Check sheet for the drawn part. Datum: minimum x, y, z corner. Units: mm. A direction names the side the tool comes from. Coordinates: 2 decimals unless noted, no trailing zeros. Loops run counter-clockwise (first coordinate to the right, second up) from the corner with the lowest first, then second, coordinate; pieces in that order, holes last. Notation, with made-up numbers: (84.25, 72.25) -> (103.25, 72.25) arc R23 ccw to (103.25, 101.25) -> close; hole circle Ø5 at (-12, 10.5). An arc over 180 degrees is marked (long way). Use CSV: the item, a comma, the result in double quotes. Start each with the question number.
1. Release check for a two-part mould opening along X. For the marked faces 3, 4 and 5 record: pulls with the +X half, pulls with the -X half, needs draft (parallel to the pull), parting line crosses it, or undercut.
2. Sectioned sample at D-D, the plane x = 37.5. Record the cut outline in (y, z), and give its area (3 significant figures).
3. Sectioned sample at A-A, the plane y = 35. Record the cut outline in (x, z).
4. Gauge pin test, flat ends, axial feed: pin 1 (8 mm diameter, centred on x = 9.5, z = 54, fed in from +Y); pin 2 (6 mm diameter, centred on y = 31.5, z = 45, fed in from -X). Record the tip position at first contact, or that the pin passes through.
5. Sectioned sample at B-B, the plane x = 30. Record the cut outline in (y, z), and give its area (3 significant figures).
6. Set-up check for the marked faces 1 and 2: record each of +Z, -Z, +X, -X, +Y, -Y from which the full face is reachable in a straight line by a thin tool's end or side.
7. Thickness scan on L1, parallel to X at y = 31, z = 38; L2, parallel to Z at x = 30, y = 1.5; L3, parallel to Y at x = 59.25, z = 45. Record the ranges inside material, lowest first.
8. Sectioned sample at C-C, the plane z = 50. Record the cut outline in (x, y), and give its area (3 significant figures).
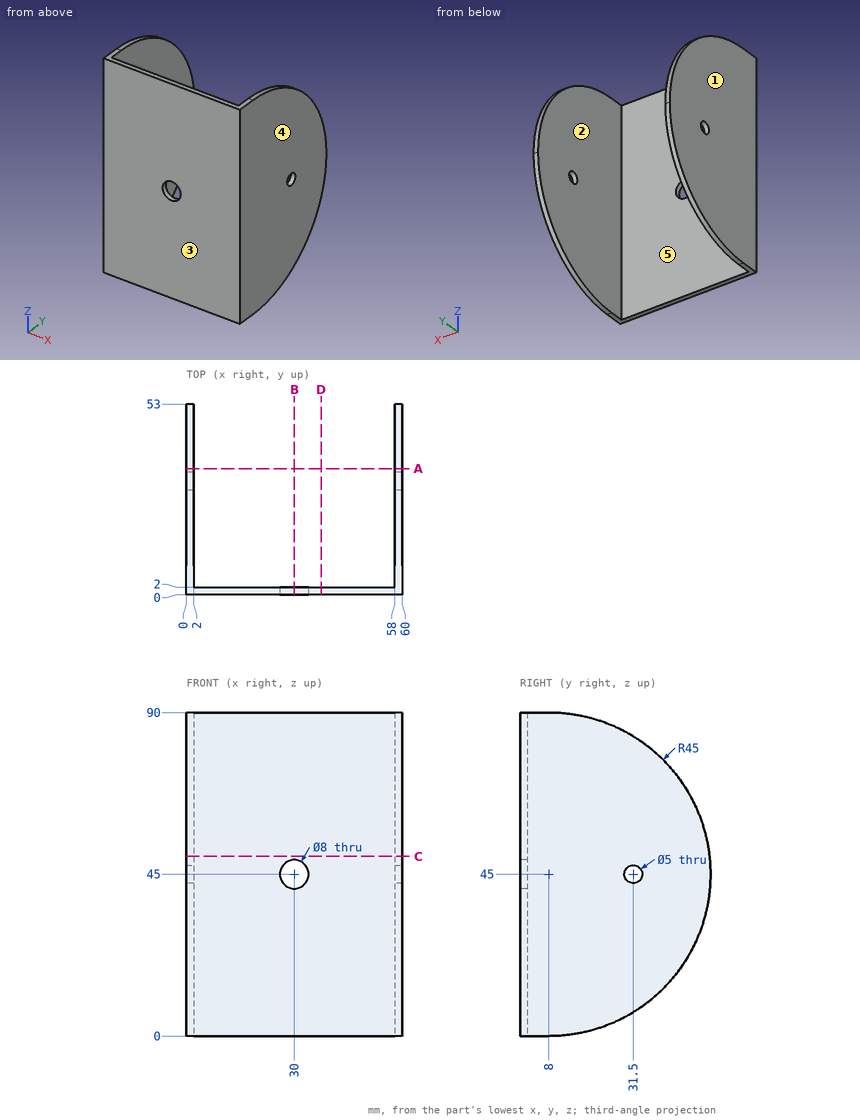
Completed:
1,face 3,"needs draft"
1,face 4,"pulls with the +X half"
1,face 5,"undercut"
2,outline,"(0, 0) -> (2, 0) -> (2, 90) -> (0, 90) -> close"
2,area,"180 mm²"
3,outline,"(0, 9) -> (2, 9) -> (2, 81) -> (0, 81) -> close; (58, 9) -> (60, 9) -> (60, 81) -> (58, 81) -> close"
4,pin 1,"y = 2"
4,pin 2,"x = 0"
5,outline,"(0, 0) -> (2, 0) -> (2, 41) -> (0, 41) -> close; (0, 49) -> (2, 49) -> (2, 90) -> (0, 90) -> close"
5,area,"164 mm²"
6,face 1,"+Z, -Z, -X, +Y, -Y"
6,face 2,"+Z, -Z, +Y"
7,L1,"0 to 2, 58 to 60"
7,L2,"0 to 41, 49 to 90"
7,L3,"0 to 29, 34 to 53"
8,outline,"(0, 0) -> (60, 0) -> (60, 52.72) -> (58, 52.72) -> (58, 2) -> (2, 2) -> (2, 52.72) -> (0, 52.72) -> close"
8,area,"323 mm²"
